Job drawing, mm, ordinate dimensions from the low corner. One solid piece. Coordinates: 2 decimals unless noted, no trailing zeros. Order: outer loops, then holes, each group sorted by start corner. A loop starts at its lowest first (then second) coordinate and runs counter-clockwise, first axis right, second up. Notation, with made-up numbers: (26.5, 16) - (72.5, 16) arc R9 cw to (72.5, 31) - close; hole circle Ø10 at (12, 17.25). An arc over 180 degrees is marked (long way). Use one line per item in the form item = value.
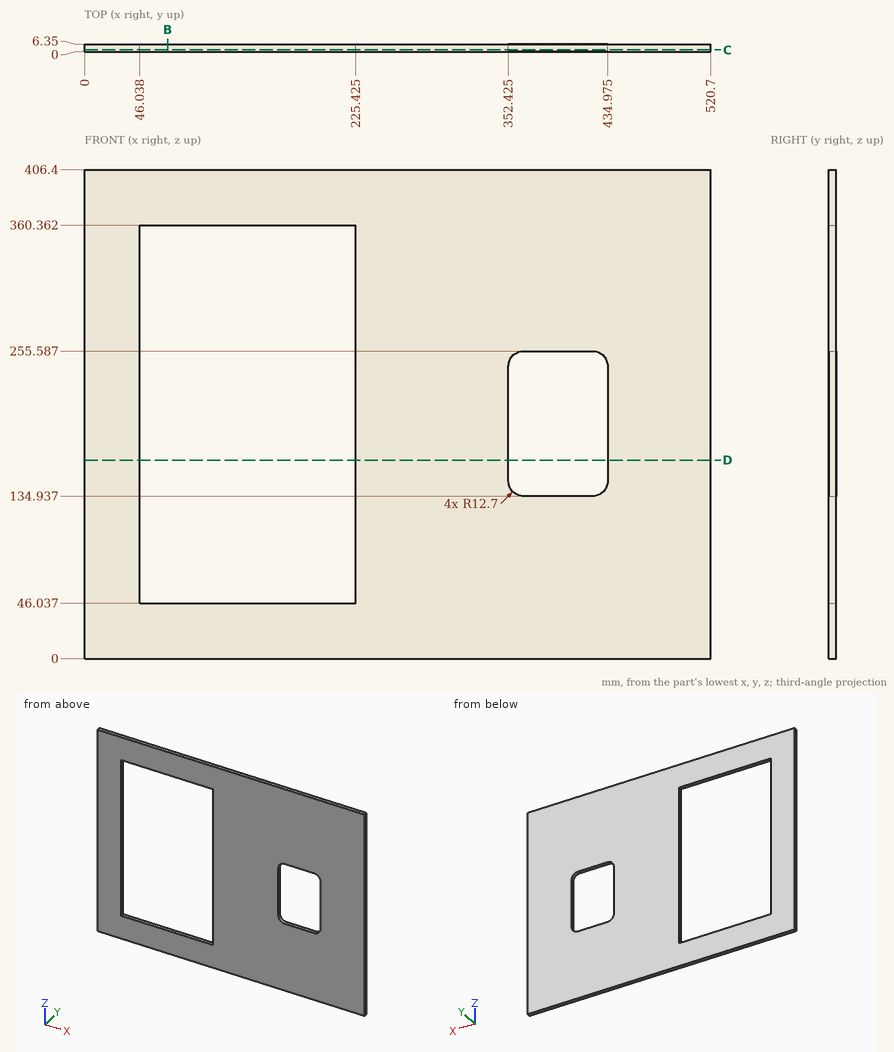
Item 1: Cut at C-C, the plane y = 1.5. Write the cut outline in (x, z) (1 decimal).
Derived:
outline = (0, 0) - (520.7, 0) - (520.7, 406.4) - (0, 406.4) - close; hole (46, 46) - (225.4, 46) - (225.4, 360.4) - (46, 360.4) - close; hole (352.4, 147.6) arc R12.7 ccw to (365.1, 134.9) - (422.3, 134.9) arc R12.7 ccw to (435, 147.6) - (435, 242.9) arc R12.7 ccw to (422.3, 255.6) - (365.1, 255.6) arc R12.7 ccw to (352.4, 242.9) - close
Item 2: Drill centre lines: line 1 (X direction, y = 5, z = 244.5) (1 decimal); line 2 (X direction, y = 6.25, z = 233.5) (1 decimal); line 3 (Z direction, x = 370.5, y = 2). Where is each one in solid material? Low to high. Write a range as [from, to].
Derived:
line_1 = [0, 46], [225.4, 352.5], [434.9, 520.7]
line_2 = [0, 46], [225.4, 352.4], [435, 520.7]
line_3 = [0, 134.94], [255.59, 406.4]
Item 3: Cut at D-D, the plane z = 165. State how many separate pieces and enclosed holes the cut face has, plus the area to 3 significant figures.
Derived:
separate_pieces = 3
enclosed_holes = 0
area = 1,640 mm²
Item 4: Cut at B-B, the plane x = 69. Write the cut outline in (y, z).
Derived:
outline = (0, 0) - (6.35, 0) - (6.35, 46.04) - (0, 46.04) - close; (0, 360.36) - (6.35, 360.36) - (6.35, 406.4) - (0, 406.4) - close
